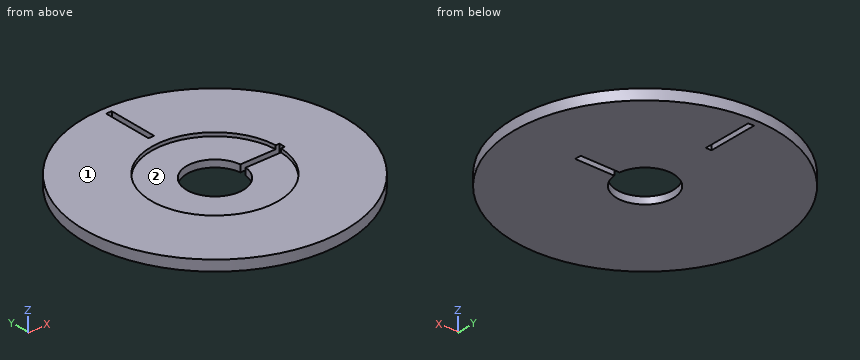
```python
from build123d import *

# Parameters (mm, degrees)
SKETCH_1_R          = 18.5
EXTRUDE_1_DEPTH     = 1.5
SKETCH_2_R          = 4
CUT_EXTRUDE_1_DEPTH = 27.205915363
SKETCH_3_R          = 9
CUT_EXTRUDE_2_DEPTH = 0.5
SKETCH_4_W          = 7
SKETCH_4_H          = 0.9
CUT_EXTRUDE_3_DEPTH = 27.205915363
SKETCH_5_W          = 0.8
SKETCH_5_H          = 7
CUT_EXTRUDE_4_DEPTH = 27.205915363


with BuildPart() as part:
    # Эскиз1 → Бобышка-Вытянуть1 (new body)
    with BuildSketch(Plane.XY):
        Circle(SKETCH_1_R)
    extrude(amount=EXTRUDE_1_DEPTH)

    # Эскиз2 → Вырез-Вытянуть1 (cut, through all)
    with BuildSketch(Plane.XY.offset(1.5)):
        Circle(SKETCH_2_R)
    extrude(amount=-CUT_EXTRUDE_1_DEPTH, mode=Mode.SUBTRACT)

    # Эскиз3 → Вырез-Вытянуть2 (cut)
    with BuildSketch(Plane.XY.offset(1.5)):
        Circle(SKETCH_3_R)
    extrude(amount=-CUT_EXTRUDE_2_DEPTH, mode=Mode.SUBTRACT)

    # Эскиз4 → Вырез-Вытянуть3 (cut, through all)
    with BuildSketch(Plane.XY.offset(1.5)):
        with Locations((6.013449427, 0)):
            Rectangle(SKETCH_4_W, SKETCH_4_H)
    extrude(amount=-CUT_EXTRUDE_3_DEPTH, mode=Mode.SUBTRACT)

    # Эскиз5 → Вырез-Вытянуть4 (cut, through all)
    with BuildSketch(Plane.XY.offset(1.5)):
        with Locations((0, 14)):
            Rectangle(SKETCH_5_W, SKETCH_5_H)
    extrude(amount=-CUT_EXTRUDE_4_DEPTH, mode=Mode.SUBTRACT)


solid = part.part
```
Build history of the part. All positions in model axes, mm. Face numbers are marked on the shaded views. Coordinates: 2 decimals unless noted, no trailing zeros. Order: outer loops, then holes, each group sorted by start corner. A loop starts at its lowest first (then second) coordinate and runs counter-clockwise, first axis right, second up. Notation, with made-up numbers: (79.5, 2.25) -> (92.5, 2.25) arc R17 cw to (92.5, 23.25) -> close; hole circle Ø11 at (34.5, 7.5). An arc over 180 degrees is marked (long way). Answer in a Markdown table with one row per item. Add a question column.
Q1. Band-saw the part on B-B, the plane x = -3. List the corners of the cut face in (y, z).
Q2. Drop flat-ended pins along their axis: pin 1 (0.6 mm diameter, centred on x = 0, z = 1, fed in from -Y); pin 2 (0.6 mm diameter, centred on x = 0, z = 0.5, fed in from +Y); pin 3 (10.5 mm diameter, centred on x = 0, y = 0, fed in from +Z). Give the stop position or say it passes through.
Q3. Band-saw the part on D-D, the plane x = 16.5. List the corners of the cut face in (y, z).
Q4. Wall check: line 1 along Y through (x, z) = (0, 0.35); line 2 along Y through (x, z) = (0, 1.25); line 3 along X through (y, z) = (4, 1.45). Give the ranges that are in metal, low to high. Write a range as [from, to].
Q5. Mould opens along Y. For the marked faces 1 and 2 say: +Y half, -Y half, draft (parallel to the pull), parting line (faces both ways), or undercut.
Q6. Band-saw the part on A-A, the plane y = 0. List the corners of the cut face in (x, z).
Q7. Band-saw the part on C-C, the plane y = -4.5. List the corners of the cut face in (x, z), then the cut area to 3 significant figures.
Answers follow:
| question | item | result |
|---|---|---|
| 1 | outline | (-18.26, 0) -> (-2.65, 0) -> (-2.65, 1) -> (-8.49, 1) -> (-8.49, 1.5) -> (-18.26, 1.5) -> close; (2.65, 0) -> (18.26, 0) -> (18.26, 1.5) -> (8.49, 1.5) -> (8.49, 1) -> (2.65, 1) -> close |
| 2 | pin 1 | y = -18.5 |
| 2 | pin 2 | y = 18.5 |
| 2 | pin 3 | z = 1 |
| 3 | outline | (-8.37, 0) -> (8.37, 0) -> (8.37, 1.5) -> (-8.37, 1.5) -> close |
| 4 | line 1 | [-18.5, -4], [4, 10.5], [17.5, 18.5] |
| 4 | line 2 | [-18.5, -9], [9, 10.5], [17.5, 18.5] |
| 4 | line 3 | [-18.06, -8.06], [8.06, 18.06] |
| 5 | face 1 | draft |
| 5 | face 2 | undercut |
| 6 | outline | (-18.5, 0) -> (-4, 0) -> (-4, 1) -> (-9, 1) -> (-9, 1.5) -> (-18.5, 1.5) -> close; (9.51, 0) -> (18.5, 0) -> (18.5, 1.5) -> (9.51, 1.5) -> close |
| 7 | outline | (-17.94, 0) -> (17.94, 0) -> (17.94, 1.5) -> (7.79, 1.5) -> (7.79, 1) -> (-7.79, 1) -> (-7.79, 1.5) -> (-17.94, 1.5) -> close |
| 7 | area | 46.0 mm^2 |
